Part model, mm, in its own coordinate system. Round coordinates to 2 decimals unless told otherwise and drop trailing zeros. Put each result on its own line as item: value. Start each with the question number.
1) Probe line 1 along X through (y, z) = (3.25, -148); line 2 along X through (y, z) = (1, -62); line 3 along X through (y, z) = (4, -45). List the from-to ranges inside material, lowest first.
2) Drop a flat-ended pin along its axis: pin 1 Ø4 at (x, z) = (-62.92, -170.47) entering from -Y (1 decimal). Give the stop position or say it passes through.
3) Pull direction Z, two halves, no side cores. Call faces 1 (the flat face through (-10, 9.652, -91)), 2 (the cylindrical face through (-2.453, 4.894, -93.336)): +Z half, -Z half, draft (parallel to the pull), parting line (faces both ways), or undercut.
```python
from build123d import *

# Parameters (mm, degrees)
SKETCH1_W           = 1567.434
SKETCH1_H           = 152.4
BOSS_EXTRUDE1_DEPTH = 9.652
SKETCH2_R           = 3.175
SKETCH2_R_2         = 13.97
CUT_EXTRUDE2_DEPTH  = 10.652


with BuildPart() as part:
    # Sketch1 → Boss-Extrude1 (new body)
    with BuildSketch(Plane(origin=(0, 0, 0), x_dir=(1, 0, 0), z_dir=(0, 1, 0))):
        with Locations((0.575131409, 106.973938621)):
            Rectangle(SKETCH1_W, SKETCH1_H)
    extrude(amount=BOSS_EXTRUDE1_DEPTH)

    # Sketch2 → Cut-Extrude2 (cut, through all)
    with BuildSketch(Plane(origin=(0, 9.652, 0), x_dir=(1, 0, 0), z_dir=(0, 1, 0))):
        with Locations((-770.441868591, 170.473938621)):
            Circle(SKETCH2_R)
        with Locations((-770.441868591, 43.473938621)):
            Circle(SKETCH2_R)
        with Locations((771.592131409, 43.473938621)):
            Circle(SKETCH2_R)
        with Locations((771.592131409, 170.473938621)):
            Circle(SKETCH2_R)
        with Locations((0.575131409, 106.973938621)):
            Circle(SKETCH2_R_2)
        with Locations((-62.924868591, 170.473938621)):
            Circle(SKETCH2_R)
        with Locations((-62.924868591, 43.473938621)):
            Circle(SKETCH2_R)
        with Locations((64.075131409, 43.473938621)):
            Circle(SKETCH2_R)
        with Locations((64.075131409, 170.473938621)):
            Circle(SKETCH2_R)
        with BuildLine():
            Line((-773.743868591, 148.502938621), (-773.743868591, 151.804938621))
            ThreePointArc((-773.743868591, 151.804938621), (-770.441868591, 155.106938621), (-767.139868591, 151.804938621))
            Line((-767.139868591, 151.804938621), (-767.139868591, 148.502938621))
            ThreePointArc((-767.139868591, 148.502938621), (-770.441868591, 145.200938621), (-773.743868591, 148.502938621))
        make_face()
        with BuildLine():
            Line((-773.743868591, 65.444938621), (-773.743868591, 62.142938621))
            ThreePointArc((-773.743868591, 62.142938621), (-770.441868591, 58.840938621), (-767.139868591, 62.142938621))
            Line((-767.139868591, 62.142938621), (-767.139868591, 65.444938621))
            ThreePointArc((-767.139868591, 65.444938621), (-770.441868591, 68.746938621), (-773.743868591, 65.444938621))
        make_face()
        with BuildLine():
            Line((774.894131409, 65.444938621), (774.894131409, 62.142938621))
            ThreePointArc((774.894131409, 62.142938621), (771.592131409, 58.840938621), (768.290131409, 62.142938621))
            Line((768.290131409, 62.142938621), (768.290131409, 65.444938621))
            ThreePointArc((768.290131409, 65.444938621), (771.592131409, 68.746938621), (774.894131409, 65.444938621))
        make_face()
        with BuildLine():
            Line((774.894131409, 148.502938621), (774.894131409, 151.804938621))
            ThreePointArc((774.894131409, 151.804938621), (771.592131409, 155.106938621), (768.290131409, 151.804938621))
            Line((768.290131409, 151.804938621), (768.290131409, 148.502938621))
            ThreePointArc((768.290131409, 148.502938621), (771.592131409, 145.200938621), (774.894131409, 148.502938621))
        make_face()
    extrude(amount=-CUT_EXTRUDE2_DEPTH, mode=Mode.SUBTRACT)


solid = part.part
```
Recorded:
1. line 1: x = -783.14 to -773.71, -767.18 to 768.33, 774.86 to 784.29
1. line 2: x = -783.14 to -773.74, -767.14 to 768.29, 774.89 to 784.29
1. line 3: x = -783.14 to -773.23, -767.66 to -65.71, -60.14 to 61.29, 66.86 to 768.81, 774.38 to 784.29
2. pin 1: passes through
3. face 1: draft
3. face 2: undercut
